Geometry check sheet. Reference: the model listing, model coordinates, mm. Face numbers are marked on the shaded views. Round coordinates to 2 decimals unless told otherwise and drop trailing zeros. Order: outer loops, then holes, each group sorted by start corner. A loop starts at its lowest first (then second) coordinate and runs counter-clockwise, first axis right, second up.
(1) Sectioned sample at D-D (z = 43). Record the boundary of the cut face in (x, y), plus the area to 3 significant figures.
(2) Sectioned sample at A-A (y = 5.5). Record the boundary of the cut face in (x, z).
(3) Release check for a two-part mould opening along Z. For the marked faces 1 and 2 record: +Z half, -Z half, draft (parallel to the pull), parting line (faces both ways), or undercut.
(4) Material ranges on line 1 along Z through (x, y) = (-4, 0.75); line 2 along Z through (x, y) = (4.5, 5.25); line 3 along X through (y, z) = (4.25, -24.5), recorded low to high.
(5) Sectioned sample at B-B (z = 0). Record the boundary of the cut face in (x, y).
(6) Sectioned sample at C-C (x = 31.5). Record the boundary of the cut face in (y, z).
(7) Go/stop test with flat-tipped pins: pin 1 (3 mm diameter, centred on y = 3.5, z = 14, fed in from -X); pin 2 (2 mm diameter, centred on x = 45.5, z = -49, fed in from +Y); pin 3 (3 mm diameter, centred on y = 1.5, z = -52.5, fed in from -X); pin 4 (4 mm diameter, centred on x = 11.5, z = -35, fed in from -Y). Record where each tip stops, or that it passes through.
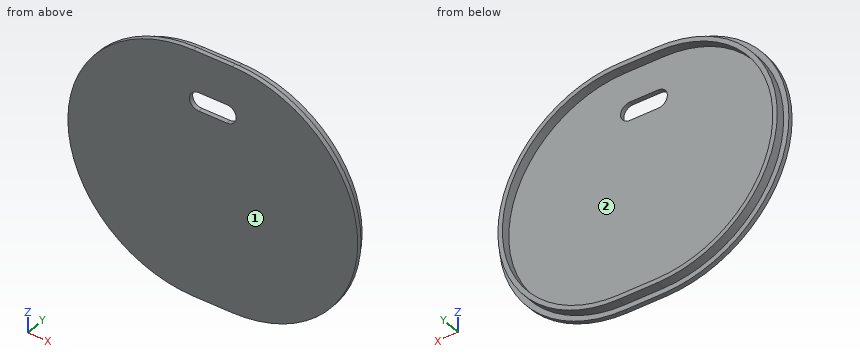
from build123d import *

# Parameters (mm, degrees)
BOSS_EXTRUDE1_DEPTH = 2.4
BOSS_EXTRUDE2_DEPTH = 4.8
CUT_EXTRUDE1_DEPTH  = 103.48316935


with BuildPart() as part:
    # Sketch1 → Boss-Extrude1 (new body)
    with BuildSketch(Plane(origin=(0, 0, 0), x_dir=(1, 0, 0), z_dir=(0, 1, 0))):
        with BuildLine():
            Line((-10.4, 67), (10.4, 67))
            ThreePointArc((10.4, 67), (77.4, 0), (10.4, -67))
            Line((10.4, -67), (-10.4, -67))
            ThreePointArc((-10.4, -67), (-77.4, 0), (-10.4, 67))
        make_face()
    extrude(amount=BOSS_EXTRUDE1_DEPTH)

    # Sketch2 → Boss-Extrude2 (add)
    with BuildSketch(Plane(origin=(0, 2.4, 0), x_dir=(1, 0, 0), z_dir=(0, 1, 0))):
        with BuildLine():
            Line((-10.4, 64.2), (10.4, 64.2))
            ThreePointArc((10.4, 64.2), (74.6, 0), (10.4, -64.2))
            Line((10.4, -64.2), (-10.4, -64.2))
            ThreePointArc((-10.4, -64.2), (-74.6, 0), (-10.4, 64.2))
        make_face()
        with BuildLine():
            Line((-10.4, 61.8), (10.4, 61.8))
            ThreePointArc((10.4, 61.8), (72.2, 0), (10.4, -61.8))
            Line((10.4, -61.8), (-10.4, -61.8))
            ThreePointArc((-10.4, -61.8), (-72.2, 0), (-10.4, 61.8))
        make_face(mode=Mode.SUBTRACT)
    extrude(amount=BOSS_EXTRUDE2_DEPTH)

    # Sketch3 → Cut-Extrude1 (cut, through all)
    with BuildSketch(Plane(origin=(0, 2.4, 0), x_dir=(1, 0, 0), z_dir=(0, 1, 0))):
        with BuildLine():
            Line((-7.5, -35), (7.5, -35))
            ThreePointArc((7.5, -35), (12.5, -40), (7.5, -45))
            Line((7.5, -45), (-7.5, -45))
            ThreePointArc((-7.5, -45), (-12.5, -40), (-7.5, -35))
        make_face()
    extrude(amount=-CUT_EXTRUDE1_DEPTH, mode=Mode.SUBTRACT)


solid = part.part
Answer below:
1. outline: (-61.78, 0) - (-11.5, 0) - (-11.5, 2.4) - (-54.79, 2.4) - (-54.79, 7.2) - (-58.07, 7.2) - (-58.07, 2.4) - (-61.78, 2.4) - close; (11.5, 0) - (61.78, 0) - (61.78, 2.4) - (58.07, 2.4) - (58.07, 7.2) - (54.79, 7.2) - (54.79, 2.4) - (11.5, 2.4) - close
1. area: 273 mm2
2. outline: (-10.4, -64.2) - (10.4, -64.2) arc R64.2 ccw to (10.4, 64.2) - (-10.4, 64.2) arc R64.2 ccw to start; hole (-10.4, -61.8) - (10.4, -61.8) arc R61.8 ccw to (10.4, 61.8) - (-10.4, 61.8) arc R61.8 ccw to start
3. face 1: draft
3. face 2: undercut
4. line 1: z = -67 to 35, 45 to 67
4. line 2: z = -64.2 to -61.8, 61.8 to 64.2
4. line 3: x = -69.74 to -67.14, 67.14 to 69.74
5. outline: (-77.4, 0) - (77.4, 0) - (77.4, 2.4) - (74.6, 2.4) - (74.6, 7.2) - (72.2, 7.2) - (72.2, 2.4) - (-72.2, 2.4) - (-72.2, 7.2) - (-74.6, 7.2) - (-74.6, 2.4) - (-77.4, 2.4) - close
6. outline: (0, -63.59) - (2.4, -63.59) - (2.4, -60.63) - (7.2, -60.63) - (7.2, -58.09) - (2.4, -58.09) - (2.4, 58.09) - (7.2, 58.09) - (7.2, 60.63) - (2.4, 60.63) - (2.4, 63.59) - (0, 63.59) - close
7. pin 1: stops at x = -76.13
7. pin 2: stops at y = 2.4
7. pin 3: stops at x = -53.85
7. pin 4: stops at y = 0
